```python
from build123d import *

# Parameters (mm, degrees)
SKETCH1_W           = 50
SKETCH1_H           = 50
BOSS_EXTRUDE1_DEPTH = 50
SKETCH2_R           = 30
BOSS_EXTRUDE2_DEPTH = 58.25
SKETCH3_R           = 7.5
CUT_EXTRUDE1_DEPTH  = 1
SKETCH4_R           = 2.4
CUT_EXTRUDE2_DEPTH  = 15
CUT_EXTRUDE3_START  = -15
SKETCH5_R           = 2.4
CUT_EXTRUDE3_DEPTH  = 15


with BuildPart() as part:
    # Sketch1 → Boss-Extrude1 (new body)
    with BuildSketch(Plane.XY):
        with Locations((25, 1.421800948)):
            Rectangle(SKETCH1_W, SKETCH1_H)
    extrude(amount=BOSS_EXTRUDE1_DEPTH)

    # Sketch2 → Boss-Extrude2 (add)
    with BuildSketch(Plane.XY.offset(50)):
        with Locations(Location((25, 0, 0), (0, 0, 146.442690238))):
            Circle(SKETCH2_R)
    extrude(amount=BOSS_EXTRUDE2_DEPTH)

    # Sketch3 → Cut-Extrude1 (cut)
    with BuildSketch(Plane(origin=(0, 0, 0), x_dir=(-1, 0, 0), z_dir=(0, 0, -1))):
        with Locations((-25, 0)):
            Circle(SKETCH3_R)
    extrude(amount=-CUT_EXTRUDE1_DEPTH, mode=Mode.SUBTRACT)

    # Sketch4 → Cut-Extrude2 (cut)
    with BuildSketch(Plane(origin=(50, 0, 0), x_dir=(0, 0, -1), z_dir=(1, 0, 0))):
        with Locations((-39, 15.421800948)):
            Circle(SKETCH4_R)
        with Locations((-11, 15.421800948)):
            Circle(SKETCH4_R)
        with Locations((-11, -12.578199052)):
            Circle(SKETCH4_R)
        with Locations((-39, -12.578199052)):
            Circle(SKETCH4_R)
    extrude(amount=-CUT_EXTRUDE2_DEPTH, mode=Mode.SUBTRACT)

    # Sketch5 → Cut-Extrude3 (cut)
    with BuildSketch(Plane.ZY.offset(CUT_EXTRUDE3_START)):
        with Locations(Location((11, 15.421800948, 0), (0, 0, 180))):
            Circle(SKETCH5_R)
        with Locations(Location((39, 15.421800948, 0), (0, 0, 180))):
            Circle(SKETCH5_R)
        with Locations(Location((39, -12.578199052, 0), (0, 0, 180))):
            Circle(SKETCH5_R)
        with Locations(Location((11, -12.578199052, 0), (0, 0, 180))):
            Circle(SKETCH5_R)
    extrude(amount=CUT_EXTRUDE3_DEPTH, mode=Mode.SUBTRACT)


solid = part.part
```
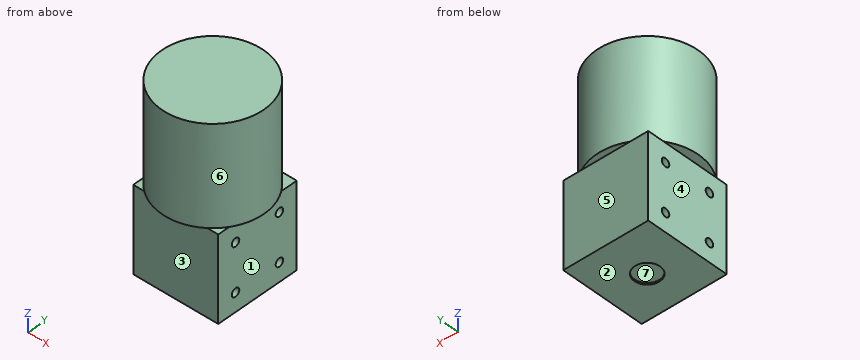
Geometry check sheet. Reference: the model listing, model coordinates, mm. Face numbers are marked on the shaded views. A direction names the side the tool comes from. Coordinates: 2 decimals unless noted, no trailing zeros. Loops run counter-clockwise (first coordinate to the right, second up) from the corner with the lowest first, then second, coordinate; pieces in that order, holes last.
Item 1: Sectioned sample at D-D, the plane x = 41.5. Record the boundary of the cut face in (y, z).
Item 2: Sectioned sample at B-B, the plane z = 11. Record the boundary of the cut face in (x, y), then the cut area to 3 significant figures.
Item 3: Thickness scan on line 1 (Y direction, x = 39, z = 11); line 2 (Y direction, x = 25, z = 0.45); line 3 (Y direction, x = 4, z = 38). Record the ranges inside material, lowest first.
Item 4: Sectioned sample at C-C, the plane x = 25. Record the boundary of the cut face in (y, z).
Item 5: Access from +Z, -Z, +X, -X, +Y, -Y to the whole of each face (thin tool, end or side, straight path). Record for the marked faces 1, 2 and 3.
Item 6: Release check for a two-part mould opening along X. For the marked faces 4, 5, 6 and 7 record: released by +X, released by -X, zero draft, split by the parting line, or undercut.
Item 7: Go/stop test with flat-tipped pins: pin 1 Ø3 at (y, z) = (15.42, 39) entering from +X; pin 2 Ø4 at (y, z) = (-20, 55.5) entering from +X; pin 3 Ø6 at (y, z) = (-12.58, 11) entering from -X; pin 4 Ø5 at (x, y) = (18, 15) entering from -Z. Record where each tip stops, or that it passes through.
Item 8: Sectioned sample at A-A, the plane y = 0. Record the boundary of the cut face in (x, z).
Check result:
1. outline: (-25.05, 50) - (-23.58, 50) - (-23.58, 0) - (26.42, 0) - (26.42, 50) - (25.05, 50) - (25.05, 108.25) - (-25.05, 108.25) - close; hole circle Ø4.8 at (-12.58, 11); hole circle Ø4.8 at (-12.58, 39); hole circle Ø4.8 at (15.42, 11); hole circle Ø4.8 at (15.42, 39)
2. outline: (0, -23.58) - (50, -23.58) - (50, -14.98) - (35, -14.98) - (35, -10.18) - (50, -10.18) - (50, 13.02) - (35, 13.02) - (35, 17.82) - (50, 17.82) - (50, 26.42) - (0, 26.42) - (0, 17.82) - (15, 17.82) - (15, 13.02) - (0, 13.02) - (0, -10.18) - (15, -10.18) - (15, -14.98) - (0, -14.98) - close
2. area: 2,210 mm2
3. line 1: y = -23.58 to -14.98, -10.18 to 13.02, 17.82 to 26.42
3. line 2: y = -23.58 to -7.5, 7.5 to 26.42
3. line 3: y = -23.58 to -14.76, -10.4 to 13.24, 17.6 to 26.42
4. outline: (-30, 50) - (-23.58, 50) - (-23.58, 0) - (-7.5, 0) - (-7.5, 1) - (7.5, 1) - (7.5, 0) - (26.42, 0) - (26.42, 50) - (30, 50) - (30, 108.25) - (-30, 108.25) - close
5. face 1: -Z, +X, +Y, -Y
5. face 2: -Z, +X, -X, +Y, -Y
5. face 3: -Z, +X, -X, -Y
6. face 4: released by -X
6. face 5: zero draft
6. face 6: split by the parting line
6. face 7: undercut
7. pin 1: stops at x = 35
7. pin 2: stops at x = 49
7. pin 3: stops at x = 0
7. pin 4: stops at z = 0
8. outline: (-5, 50) - (0, 50) - (0, 0) - (17.5, 0) - (17.5, 1) - (32.5, 1) - (32.5, 0) - (50, 0) - (50, 50) - (55, 50) - (55, 108.25) - (-5, 108.25) - close
